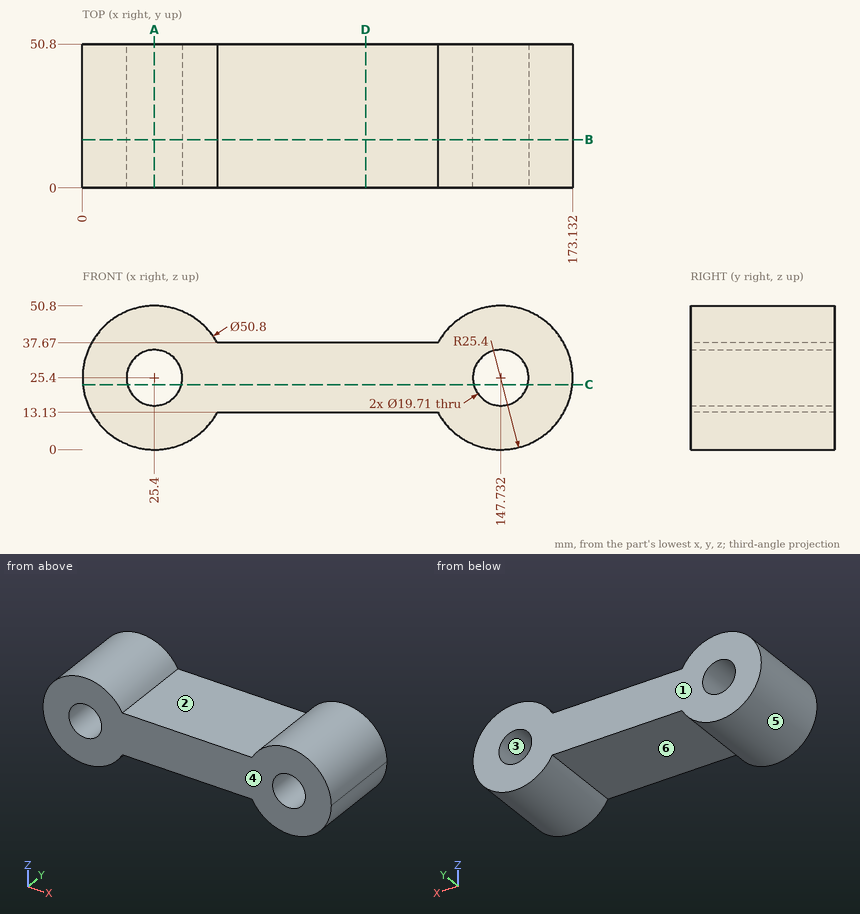
Verification items for this drawing (mm, ordinates from the low corner). A direction names the side the tool comes from. Coordinates: 2 decimals unless noted, no trailing zeros. Write each loop counter-clockwise with the first axis right and the second up, starting at its lowest first coordinate (ties: lowest second). Pieces come first, ordered by that corner, then holes. Notation, with made-up numbers: M 86.25,10 L 135.25,10 A17 ccw 135.25,37 Z; hole C 59.5,65.25 d4. An arc over 180 degrees is marked long. Answer as a JSON object with one key per item and string values.
1. Go/stop test with flat-tipped pins: pin 1 Ø12 at (y, z) = (21.5, 8) entering from -X; pin 2 Ø1 at (x, y) = (119.5, 18.5) entering from +Z; pin 3 Ø2 at (x, y) = (30, 17) entering from +Z. Record where each tip stops, or that it passes through.
Answers below:
{"pin 1": "stops at x = 2.7", "pin 2": "stops at z = 37.67", "pin 3": "stops at z = 50.54"}
2. Section check B-B, the plane y = 17. Enter the section's corners in (x, z) (1 decimal).
Answers below:
{"outline": "M 47.6,13.1 L 125.5,13.1 A25.4 ccw long 125.5,37.7 L 47.6,37.7 A25.4 ccw long Z; hole C 25.4,25.4 d19.7; hole C 147.7,25.4 d19.7"}
3. Section check A-A, the plane x = 25.4. Enter the section's corners in (y, z) (1 decimal).
Answers below:
{"outline": "M 0,0 L 50.8,0 L 50.8,15.5 L 0,15.5 Z; M 0,35.3 L 50.8,35.3 L 50.8,50.8 L 0,50.8 Z"}
4. Section check D-D, the plane x = 100. Enter the section's corners in (y, z), plus the area to 3 significant figures.
Answers below:
{"outline": "M 0,13.13 L 50.8,13.13 L 50.8,37.67 L 0,37.67 Z", "area": "1,250 mm²"}
5. Tool access check on the marked faces 1 and 2. Record the directions out of +Z, -Z, +X, -X, +Y, -Y that give a thin tool (end or side, any length) a straight path to the whole face; none if there is none.
Answers below:
{"face 1": "+Z, -Z, +X, -X, +Y", "face 2": "+Z, +Y, -Y"}
6. Section check C-C, the plane z = 23. Enter the section's corners in (x, y).
Answers below:
{"outline": "M 0.11,0 L 15.84,0 L 15.84,50.8 L 0.11,50.8 Z; M 34.96,0 L 138.17,0 L 138.17,50.8 L 34.96,50.8 Z; M 157.29,0 L 173.02,0 L 173.02,50.8 L 157.29,50.8 Z"}
7. Scan lines: L1, parallel to X at y = 31, z = 25 (1 decimal); L2, parallel to Z at x = 25.4, y = 34.5 (1 decimal); L3, parallel to X at y = 13, z = 19.5 (1 decimal). Record each from-to range of solid material in increasing order.
Answers below:
{"L1": "x = 0 to 15.6, 35.2 to 137.9, 157.6 to 173.1", "L2": "z = 0 to 15.5, 35.3 to 50.8", "L3": "x = 0.7 to 17.5, 33.3 to 139.8, 155.6 to 172.4"}
8. Draft check along Z on the marked faces 3, 4, 5 and 6. Enter one of: released by +Z, released by -Z, zero draft, split by the parting line, or undercut.
Answers below:
{"face 3": "undercut", "face 4": "zero draft", "face 5": "split by the parting line", "face 6": "released by -Z"}
